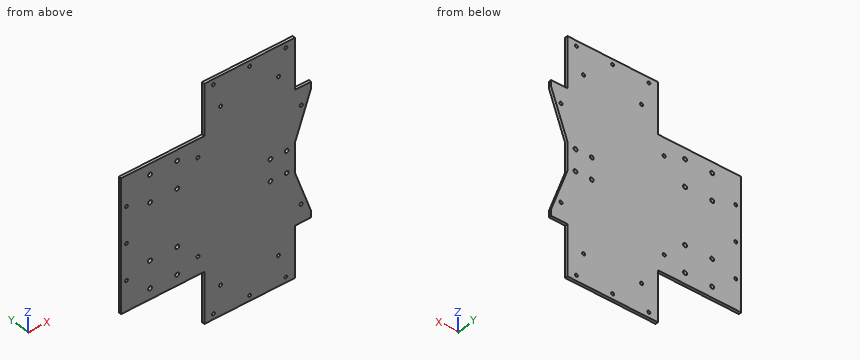
from build123d import *

# Parameters (mm, degrees)
EXTRUDE_1_DEPTH     = 3
SKETCH_2_R          = 2.15
SKETCH_2_R_2        = 1.65
SKETCH_2_R_3        = 2.2
CUT_EXTRUDE_1_DEPTH = 10
SKETCH_3_R          = 1.75
CUT_EXTRUDE_2_DEPTH = 4.5


with BuildPart() as part:
    # 草图1 → 凸台-拉伸1 (new body)
    with BuildSketch(Plane(origin=(0, 0, 0), x_dir=(1, 0, 0), z_dir=(0, 1, 0))):
        Polygon((-105, -73.5), (-13, -73.5), (-13, -130), (87, -130), (87, -73.5), (105, -73.5), (105, -66.5), (87, -16), (87, 16), (105, 66.5), (105, 73.5), (87, 73.5), (87, 130), (-13, 130), (-13, 73.5), (-105, 73.5), align=None)
    extrude(amount=EXTRUDE_1_DEPTH)

    # 草图2 → 切除-拉伸1 (cut)
    with BuildSketch(Plane.XZ):
        with Locations(Location((78, -12, 0), (0, 0, 270))):
            Circle(SKETCH_2_R)
        with Locations(Location((60, -12, 0), (0, 0, 270))):
            Circle(SKETCH_2_R)
        with Locations(Location((60, 12, 0), (0, 0, 90))):
            Circle(SKETCH_2_R)
        with Locations(Location((78, 12, 0), (0, 0, 90))):
            Circle(SKETCH_2_R)
        with Locations(Location((-3, -124, 0), (0, 0, 270))):
            Circle(SKETCH_2_R_2)
        with Locations(Location((37, -124, 0), (0, 0, 270))):
            Circle(SKETCH_2_R_2)
        with Locations(Location((77, -124, 0), (0, 0, 270))):
            Circle(SKETCH_2_R_2)
        with Locations(Location((77, 124, 0), (0, 0, 90))):
            Circle(SKETCH_2_R_2)
        with Locations(Location((37, 124, 0), (0, 0, 90))):
            Circle(SKETCH_2_R_2)
        with Locations(Location((-3, 124, 0), (0, 0, 90))):
            Circle(SKETCH_2_R_2)
        with Locations(Location((-99, -40, 0), (0, 0, 270))):
            Circle(SKETCH_2_R_2)
        with Locations(Location((-99, 40, 0), (0, 0, 90))):
            Circle(SKETCH_2_R_2)
        with Locations(Location((-73, 61.5, 0), (0, 0, 270))):
            Circle(SKETCH_2_R_3)
        with Locations(Location((-73, 31.5, 0), (0, 0, 270))):
            Circle(SKETCH_2_R_3)
        with Locations(Location((-43, 61.5, 0), (0, 0, 90))):
            Circle(SKETCH_2_R_3)
        with Locations(Location((-43, 31.5, 0), (0, 0, 90))):
            Circle(SKETCH_2_R_3)
        with Locations(Location((-43, -31.5, 0), (0, 0, 270))):
            Circle(SKETCH_2_R_3)
        with Locations(Location((-43, -61.5, 0), (0, 0, 270))):
            Circle(SKETCH_2_R_3)
        with Locations(Location((-73, -31.5, 0), (0, 0, 90))):
            Circle(SKETCH_2_R_3)
        with Locations(Location((-73, -61.5, 0), (0, 0, 90))):
            Circle(SKETCH_2_R_3)
        with Locations(Location((-99, 0, 0), (0, 0, 270))):
            Circle(SKETCH_2_R_2)
    extrude(amount=-CUT_EXTRUDE_1_DEPTH, mode=Mode.SUBTRACT)

    # 草图3 → 切除-拉伸2 (cut)
    with BuildSketch(Plane(origin=(0, 3, 0), x_dir=(1, 0, 0), z_dir=(0, 1, 0))):
        with Locations(Location((-20.002701991, 53.5, 0), (0, 0, 270))):
            Circle(SKETCH_3_R)
        with Locations(Location((4.997298009, 96.801270189, 0), (0, 0, 270))):
            Circle(SKETCH_3_R)
        with Locations(Location((69.002701991, 96.801270189, 0), (0, 0, 270))):
            Circle(SKETCH_3_R)
        with Locations(Location((94.002701991, 53.5, 0), (0, 0, 270))):
            Circle(SKETCH_3_R)
        with Locations(Location((94.002701991, -53.5, 0), (0, 0, 270))):
            Circle(SKETCH_3_R)
        with Locations(Location((69.002701991, -96.801270189, 0), (0, 0, 270))):
            Circle(SKETCH_3_R)
        with Locations(Location((4.997298009, -96.801270189, 0), (0, 0, 270))):
            Circle(SKETCH_3_R)
        with Locations(Location((-20.002701991, -53.5, 0), (0, 0, 270))):
            Circle(SKETCH_3_R)
    extrude(amount=-CUT_EXTRUDE_2_DEPTH, mode=Mode.SUBTRACT)


solid = part.part
Read the model definition and answer for the solid it produces. Units are mm, in the model's axes. Round coordinates to 2 decimals unless told otherwise and drop trailing zeros. Loops run counter-clockwise (first coordinate to the right, second up) from the corner with the lowest first, then second, coordinate; pieces in that order, holes last.
Q1. Section A-A on z = -6 is taken. Write down the section's boundary in (x, y).
Q2. Consider probe 1 along Z at (x, y) = (-99, 1.45); probe 2 along X at (y, z) = (2, 124); probe 3 along X at (y, z) = (2.2, -12). Determine where each line is inside the solid, lowest interval first.
Q3. Each of these flat-tipped pins is pushed along its axis until it touches: pin 1 (2 mm diameter, centred on x = -3, z = 124, fed in from -Y); pin 2 (4 mm diameter, centred on x = 5, z = -96.8, fed in from -Y); pin 3 (0.9 mm diameter, centred on y = 1, z = -2, fed in from +X). Where does it stop, or does it pass through?
Q4. Section C-C on y = 1.9 is taken. Give the number of separate pieces and of enclosed holes in the cut face, and give its area (3 significant figures).
Q5. Section B-B on x = -88.5 is taken. Write down the section's boundary in (y, z).
Output:
1. outline: (-105, 0) - (87, 0) - (87, 3) - (-105, 3) - close
2. probe 1: z = -73.5 to -41.65, -38.35 to -1.65, 1.65 to 38.35, 41.65 to 73.5
2. probe 2: x = -13 to -4.65, -1.35 to 35.35, 38.65 to 75.35, 78.65 to 87
2. probe 3: x = -105 to 57.85, 62.15 to 75.85, 80.15 to 87
3. pin 1: passes through
3. pin 2: stops at y = 0
3. pin 3: stops at x = 87
4. separate pieces: 1
4. enclosed holes: 29
4. area: 40,400 mm2
5. outline: (0, -73.5) - (3, -73.5) - (3, 73.5) - (0, 73.5) - close
